from build123d import *

# Parameters (mm, degrees)
EXTRUDE_1_DEPTH = 5


with BuildPart() as part:
    # 草图1 → 凸台-拉伸1 (new body)
    with BuildSketch(Plane.XY):
        with BuildLine():
            ThreePointArc((0, 144), (-144, 0), (0, -144))
            ThreePointArc((0, -144), (144, 0), (0, 144))
        make_face()
        with BuildLine():
            ThreePointArc((31.004898177, 121.09375), (0, 125), (-31.004898177, 121.09375))
            ThreePointArc((-31.004898177, 121.09375), (-49.607837082, 93.75), (-24.803918541, 71.875))
            ThreePointArc((-24.803918541, 71.875), (-21.678918541, 72.071081459), (-18.602938906, 72.65625))
            ThreePointArc((-18.602938906, 72.65625), (0, 75), (18.602938906, 72.65625))
            ThreePointArc((18.602938906, 72.65625), (21.678918541, 72.071081459), (24.803918541, 71.875))
            ThreePointArc((24.803918541, 71.875), (49.607837082, 93.75), (31.004898177, 121.09375))
        make_face(mode=Mode.SUBTRACT)
        with BuildLine():
            ThreePointArc((0, -13.5), (13.5, 0), (0, 13.5))
            ThreePointArc((0, 13.5), (-13.5, 0), (0, -13.5))
        make_face(mode=Mode.SUBTRACT)
        with BuildLine():
            ThreePointArc((17.5, -2), (19.5, 0), (17.5, 2))
            ThreePointArc((17.5, 2), (15.5, 0), (17.5, -2))
        make_face(mode=Mode.SUBTRACT)
        with BuildLine():
            ThreePointArc((0, -19.5), (2, -17.5), (0, -15.5))
            ThreePointArc((0, -15.5), (-2, -17.5), (0, -19.5))
        make_face(mode=Mode.SUBTRACT)
        with BuildLine():
            ThreePointArc((-17.5, -2), (-15.5, 0), (-17.5, 2))
            ThreePointArc((-17.5, 2), (-19.5, 0), (-17.5, -2))
        make_face(mode=Mode.SUBTRACT)
        with BuildLine():
            ThreePointArc((0, 15.5), (2, 17.5), (0, 19.5))
            ThreePointArc((0, 19.5), (-2, 17.5), (0, 15.5))
        make_face(mode=Mode.SUBTRACT)
    extrude(amount=EXTRUDE_1_DEPTH)


solid = part.part
For this review, take the finished solid that the model builds, in its own axes (mm). Round coordinates to 2 decimals unless told otherwise and drop trailing zeros. Write each loop counter-clockwise with the first axis right and the second up, starting at its lowest first coordinate (ties: lowest second). Pieces come first, ordered by that corner, then holes. Notation, with made-up numbers: M 6.25,28 L 51.25,28 A10 ccw 51.25,43 Z; hole C 18.25,85.25 d10. An arc over 180 degrees is marked long. Write item = value, one per line. Start each with the question number.
(1) Clearance check with flat-ended pins moving along their axes: pin 1 Ø1 at (x, z) = (69.5, 1) entering from +Y; pin 2 Ø3 at (y, z) = (-75.5, 3) entering from +X; pin 3 Ø1.5 at (y, z) = (70, 2.5) entering from +X; pin 4 Ø2.5 at (x, y) = (0, -17.5) entering from +Z. State where each tip first meets the part, or that it passes through.
(2) For line 1 along X through (y, z) = (0, 2.4); line 2 along Y through (x, z) = (17.5, 2.8); line 3 along Y through (x, z) = (9, 2.9), list the stretches that pass through material, from the lowest coordinate up.
(3) We need section B-B (x = -43.5). Give the boundary of the cut face in (y, z).
(4) We need section C-C (x = 71.5). Give the boundary of the cut face in (y, z) (3 decimals).
(5) We need section D-D (y = 25). Give the boundary of the cut face in (x, z), then the cut area to 3 significant figures.
(6) We need section A-A (z = 2.45). Give the boundary of the cut face in (x, y) (3 decimals), then the cut area to 3 significant figures.
(7) The part is to be moulded in two halves that separate along Y. For faces 1 (the face through (-2, -30, 5)), 2 (the face through (13.18, -2.93, 2.46)), 3 (the face through (43.25, -137.35, 2.46)), say which applies: +Y half, -Y half, draft (parallel to the pull), parting line (faces both ways), or undercut.
Results found:
q1.pin_1 = 126.39
q1.pin_2 = 123.53
q1.pin_3 = 126.26
q1.pin_4 = through
q2.line_1 = -144 to -19.5, -15.5 to -13.5, 13.5 to 15.5, 19.5 to 144
q2.line_2 = -142.93 to -2, 2 to 72.93, 123.77 to 142.93
q2.line_3 = -143.72 to -10.06, 10.06 to 74.46, 124.68 to 143.72
q3.outline = M -137.27,0 L 80.28,0 L 80.28,5 L -137.27,5 Z; M 113.47,0 L 137.27,0 L 137.27,5 L 113.47,5 Z
q4.outline = M -124.995,0 L 124.995,0 L 124.995,5 L -124.995,5 Z
q5.outline = M -141.81,0 L 141.81,0 L 141.81,5 L -141.81,5 Z
q5.area = 1,420 mm²
q6.outline = C 0,0 d288; hole M -31.005,121.094 A25 ccw -18.603,72.656 A75 cw 18.603,72.656 A25 ccw 31.005,121.094 A125 ccw Z; hole C -17.5,0 d4; hole C 0,0 d27; hole C 0,-17.5 d4; hole C 0,17.5 d4; hole C 17.5,0 d4
q6.area = 60,100 mm²
q7.face_1 = draft
q7.face_2 = undercut
q7.face_3 = parting line
